```python
from build123d import *

# Parameters (mm, degrees)
RESSALTO_EXTRUS_O1_DEPTH = 4
RESSALTO_EXTRUS_O2_DEPTH = 4
ESBO_O2_W                = 30
ESBO_O2_H                = 4
RESSALTO_EXTRUS_O3_DEPTH = 5
RESSALTO_EXTRUS_O4_DEPTH = 5
ESBO_O5_W                = 22
ESBO_O5_H                = 1
CORTE_EXTRUS_O2_DEPTH    = 35
CORTE_EXTRUS_O3_DEPTH    = 10
ESBO_O9_W                = 23
ESBO_O9_H                = 14.5
RESSALTO_EXTRUS_O5_DEPTH = 3.2
ESBO_O4_W                = 0.5
ESBO_O4_H                = 20
CORTE_EXTRUS_O4_DEPTH    = 4
ESBO_O11_R               = 1.5
ESBO_O12_R               = 1.3
ESBO_O11_4_R             = 1.5
ESBO_O12_4_R             = 1.3


with BuildPart() as part:
    # Esbo_o1 → Ressalto-extrus_o1 (new body)
    with BuildSketch(Plane(origin=(0, 0, 0), x_dir=(1, 0, 0), z_dir=(0, 1, 0))):
        with BuildLine():
            ThreePointArc((-4.5, -7.5), (-5.7, -6.3), (-6.9, -7.5))
            Line((-6.9, -7.5), (-5.7, -7.5))
            Line((-5.7, -7.5), (-4.5, -7.5))
        make_face()
        with BuildLine():
            Line((-5.7, -7.5), (-6.9, -7.5))
            ThreePointArc((-6.9, -7.5), (-5.7, -8.7), (-4.5, -7.5))
            Line((-4.5, -7.5), (-5.7, -7.5))
        make_face()
        with BuildLine():
            ThreePointArc((7, -7.5), (8.2, -8.7), (9.4, -7.5))
            Line((9.4, -7.5), (8.2, -7.5))
            Line((8.2, -7.5), (7, -7.5))
        make_face()
        with BuildLine():
            Line((8.2, -7.5), (9.4, -7.5))
            ThreePointArc((9.4, -7.5), (8.2, -6.3), (7, -7.5))
            Line((7, -7.5), (8.2, -7.5))
        make_face()
    extrude(amount=RESSALTO_EXTRUS_O1_DEPTH)



with BuildPart() as body_2:
    # Esbo_o1_3 → Ressalto-extrus_o2 (new body)
    with BuildSketch(Plane(origin=(0, 0, 0), x_dir=(1, 0, 0), z_dir=(0, 1, 0))):
        Polygon((-13, -10), (-13, -9), (-13, -7.5), (-13, 10), (-11.5, 10), (13, 10), (13, -7.5), (13, -9), (13, -10), (15, -10), (15, 10), (15, 12), (13, 12), (-13, 12), (-15, 12), (-15, 10), (-15, -10), align=None)
    extrude(amount=RESSALTO_EXTRUS_O2_DEPTH)


with BuildPart() as part_1:
    add(part.part)

    add(body_2.part)  # Ressalto-extrus_o3 merges body 2
    # Esbo_o2 → Ressalto-extrus_o3 (add)
    with BuildSketch(Plane(origin=(0, 4, 0), x_dir=(1, 0, 0), z_dir=(0, 1, 0))):
        with Locations((0, -8)):
            Rectangle(ESBO_O2_W, ESBO_O2_H)
    extrude(amount=RESSALTO_EXTRUS_O3_DEPTH)

    # Esbo_o3 → Ressalto-extrus_o4 (add)
    with BuildSketch(Plane(origin=(0, 4, 0), x_dir=(1, 0, 0), z_dir=(0, 1, 0))):
        Polygon((-11.5, 8.5), (11.5, 8.5), (11.5, -6), (13, -6), (13, 10), (-13, 10), (-13, -6), (-11.5, -6), align=None)
        Polygon((13, 10), (13, -6), (15, -6), (15, 12), (-15, 12), (-15, -6), (-13, -6), (-13, 10), align=None)
    extrude(amount=RESSALTO_EXTRUS_O4_DEPTH)

    # Esbo_o5 → Corte-extrus_o2 (cut)
    with BuildSketch(Plane.ZY.offset(15)):
        with Locations((-1, 0.5)):
            Rectangle(ESBO_O5_W, ESBO_O5_H)
    extrude(amount=-CORTE_EXTRUS_O2_DEPTH, mode=Mode.SUBTRACT)

    # Esbo_o8 → Corte-extrus_o3 (cut)
    with BuildSketch(Plane.XZ.offset(-1)):
        with BuildLine():
            Line((-15, -12), (-13, -12))
            ThreePointArc((-13, -12), (-14.414213562, -11.414213562), (-15, -10))
            Line((-15, -10), (-15, -12))
        make_face()
        with BuildLine():
            ThreePointArc((15, -10), (14.414213562, -11.414213562), (13, -12))
            Line((13, -12), (15, -12))
            Line((15, -12), (15, -10))
        make_face()
    extrude(amount=-CORTE_EXTRUS_O3_DEPTH, mode=Mode.SUBTRACT)

    # Esbo_o9 → Ressalto-extrus_o5 (add)
    with BuildSketch(Plane(origin=(0, 9, 0), x_dir=(1, 0, 0), z_dir=(0, 1, 0))):
        with BuildLine():
            Line((13, 12), (-13, 12))
            ThreePointArc((-13, 12), (-14.414213562, 11.414213562), (-15, 10))
            Line((-15, 10), (-15, -10))
            Line((-15, -10), (15, -10))
            Line((15, -10), (15, 10))
            ThreePointArc((15, 10), (14.414213562, 11.414213562), (13, 12))
        make_face()
        with Locations((0, 1.25)):
            Rectangle(ESBO_O9_W, ESBO_O9_H, mode=Mode.SUBTRACT)
    extrude(amount=RESSALTO_EXTRUS_O5_DEPTH)

    # Esbo_o4 → Corte-extrus_o4 (cut)
    with BuildSketch(Plane.XZ):
        with Locations((-13.25, 0)):
            Rectangle(ESBO_O4_W, ESBO_O4_H)
        with Locations((13.25, 0)):
            Rectangle(ESBO_O4_W, ESBO_O4_H)
    extrude(amount=-CORTE_EXTRUS_O4_DEPTH, mode=Mode.SUBTRACT)

    # Esbo_o11 → Loft4 section 0
    with BuildSketch(Plane.XZ.offset(-4)):
        with Locations((-5.7, 7.5)):
            Circle(ESBO_O11_R)
    # Esbo_o12 → Loft4 section 1
    with BuildSketch(Plane(origin=(0, 3, 0), x_dir=(-1, 0, 0), z_dir=(0, -1, 0))):
        with Locations((5.7, -7.5)):
            Circle(ESBO_O12_R)
    loft()

    # Esbo_o11_4 → Loft5 section 0
    with BuildSketch(Plane.XZ.offset(-4)):
        with Locations((8.2, 7.5)):
            Circle(ESBO_O11_4_R)
    # Esbo_o12_4 → Loft5 section 1
    with BuildSketch(Plane(origin=(0, 3, 0), x_dir=(-1, 0, 0), z_dir=(0, -1, 0))):
        with Locations((-8.2, -7.5)):
            Circle(ESBO_O12_4_R)
    loft()


solid = part_1.part
```
Model file for the job. Use its own axes, mm. A direction names the side the tool comes from. Coordinates: 2 decimals unless noted, no trailing zeros. Loops run counter-clockwise (first coordinate to the right, second up) from the corner with the lowest first, then second, coordinate; pieces in that order, holes last. Notation, with made-up numbers: (67.25, 40) - (82.25, 40) arc R33 cw to (82.25, 74) - close; hole circle Ø11 at (-4.75, 35). An arc over 180 degrees is marked (long way). Write item = value, one per line. Start each with the question number.
Item 1: 3-axis set-ups, long thin cutter, end or side, ignore diameter. For faces 1 (the face through (7.316, 1.986, 6.689)), 2 (the face through (11.5, 8, -1)), 3 (the face through (8, 1, 7)): which of +Z, -Z, +X, -X, +Y, -Y reach the whole face in a straight line?
Item 2: Drop a flat-ended pin along its axis: pin 1 Ø4 at (x, z) = (-2.5, 5) entering from +Y. Give the stop position or say it passes through.
Item 3: Saw through at C-C, the plane z = 5.5. List the corners of the cut face in (x, y).
Item 4: Wall check: probe 1 along Z at (x, y) = (-8, 6.25); probe 2 along X at (y, z) = (3.25, -6.5); probe 3 along X at (y, z) = (7.75, 0.25). Give the ranges that are in metal, low to high. Write a range as [from, to].
Item 5: Saw through at B-B, the plane y = 2.25. List the corners of the cut face in (x, z), then the cut area to 3 significant figures.
Item 6: Pull direction Z, two halves, no side cores. Call faces 4 (the face through (0, 8, 10)), 5 (the face through (13.5, 2, 0)), 6 (the face through (0, 8, 6)): +Z half, -Z half, draft (parallel to the pull), parting line (faces both ways), or undercut.
Item 7: Saw through at A-A, the plane x = -1.75. List the corners of the cut face in (y, z).
Item 8: Saw through at D-D, the plane y = 6.75. List the corners of the cut face in (x, z).
Answers:
q1.face_1 = -Y
q1.face_2 = +Y, -Y
q1.face_3 = +Z, -Z, +X, -X, -Y
q2.pin_1 = 12.2
q3.outline = (-15, 1) - (-13.5, 1) - (-13.5, 4) - (-11.5, 4) - (-11.5, 12.2) - (-15, 12.2) - close; (11.5, 4) - (13.5, 4) - (13.5, 1) - (15, 1) - (15, 12.2) - (11.5, 12.2) - close
q4.probe_1 = [-12, -8.5], [6, 10]
q4.probe_2 = [-15, -13.5], [13.5, 15]
q4.probe_3 = [-15, -11.5], [11.5, 15]
q5.outline = (-15, -10) arc R2 ccw to (-13, -12) - (13, -12) arc R2 ccw to (15, -10) - (15, 10) - (13.5, 10) - (13.5, -10) - (-13.5, -10) - (-13.5, 10) - (-15, 10) - close; circle Ø2.4 at (-5.7, 7.5); circle Ø2.4 at (8.2, 7.5)
q5.area = 127 mm2
q6.face_4 = +Z half
q6.face_5 = draft
q6.face_6 = undercut
q7.outline = (1, -12) - (12.2, -12) - (12.2, -8.5) - (4, -8.5) - (4, -10) - (1, -10) - close; (4, 6) - (12.2, 6) - (12.2, 10) - (4, 10) - close
q8.outline = (-15, -10) arc R2 ccw to (-13, -12) - (13, -12) arc R2 ccw to (15, -10) - (15, 10) - (-15, 10) - close; hole (-11.5, -8.5) - (11.5, -8.5) - (11.5, 6) - (-11.5, 6) - close
